from build123d import *

# Parameters (mm, degrees)
SALIENTE_EXTRUIR1_DEPTH      = 2.4
CROQUIS2_W                   = 0.6
CROQUIS2_H                   = 0.6
SALIENTE_EXTRUIR2_DEPTH      = 6
SALIENTE_EXTRUIR3_DEPTH      = 3
SALIENTE_EXTRUIR3_DEPTH_BACK = 2
CROQUIS3_W                   = 0.6
CROQUIS3_H                   = 0.6


with BuildPart() as part:
    # Croquis1 → Saliente-Extruir1 (new body)
    with BuildSketch(Plane(origin=(0, 0, 0), x_dir=(1, 0, 0), z_dir=(0, 1, 0))):
        Polygon((-1, 1.25), (1, 1.25), (1.25, 1), (1.25, -1), (1, -1.25), (-1, -1.25), (-1.25, -1), (-1.25, 1), align=None)
    extrude(amount=SALIENTE_EXTRUIR1_DEPTH)

    # Croquis2 → Saliente-Extruir2 (add)
    with BuildSketch(Plane(origin=(0, 2.4, 0), x_dir=(1, 0, 0), z_dir=(0, 1, 0))):
        Rectangle(CROQUIS2_W, CROQUIS2_H)
    extrude(amount=SALIENTE_EXTRUIR2_DEPTH)

    # Croquis3 → Saliente-Extruir3 (add, two sides: drawn at the far end of the back side and taken through both)
    with BuildSketch(Plane.XZ.offset(-SALIENTE_EXTRUIR3_DEPTH_BACK)):
        Rectangle(CROQUIS3_W, CROQUIS3_H)
    extrude(amount=SALIENTE_EXTRUIR3_DEPTH + SALIENTE_EXTRUIR3_DEPTH_BACK)


solid = part.part
Input: part model. Units: mm. Frame: model coordinates. Give positions to 0.01 mm unless a question says otherwise; leave off trailing zeros. Loops run counter-clockwise (first coordinate to the right, second up) from the corner with the lowest first, then second, coordinate; pieces in that order, holes last. Notation, with made-up numbers: (63.25, 8.25) - (120.25, 8.25) arc R31 cw to (120.25, 36.25) - close; hole circle Ø11 at (-12, 77). An arc over 180 degrees is marked (long way). Use CSV: the item, a comma, the result in double quotes. Start each with the question number.
Item 1: Contact query for flat-ended pins moving along their axis: P1, Ø0.7, axis at y = 6, z = 0, coming from the -X side; P2, Ø0.5, axis at y = -1.5, z = 0, coming from the +X side; P3, Ø0.5, axis at x = 0, y = 5.5, coming from the -Z side. Output: stop coordinate, or through.
Item 2: Line query: line 1 (X direction, y = 8.25, z = -0.05); line 2 (Y direction, x = 0.4, z = -0.6). Output: solid intervals per line, ascending.
Item 3: Section B-B on z = 0.55. Return loops of the section in (x, y), then the cut area to 3 significant figures.
Item 4: Section A-A on x = -0.15. Return loops of the section in (y, z), then the cut area to 3 significant figures.
Item 5: Section C-C on y = 5.25. Return loops of the section in (x, z), then the cut area to 3 significant figures.
Ans:
1,P1,"stops at x = -0.3"
1,P2,"stops at x = 0.3"
1,P3,"stops at z = -0.3"
2,line 1,"x = -0.3 to 0.3"
2,line 2,"y = 0 to 2.4"
3,outline,"(-1.25, 0) - (1.25, 0) - (1.25, 2.4) - (-1.25, 2.4) - close"
3,area,"6.00 mm2"
4,outline,"(-3, -0.3) - (0, -0.3) - (0, -1.25) - (2.4, -1.25) - (2.4, -0.3) - (8.4, -0.3) - (8.4, 0.3) - (2.4, 0.3) - (2.4, 1.25) - (0, 1.25) - (0, 0.3) - (-3, 0.3) - close"
4,area,"11.4 mm2"
5,outline,"(-0.3, -0.3) - (0.3, -0.3) - (0.3, 0.3) - (-0.3, 0.3) - close"
5,area,"0.360 mm2"
